```python
from build123d import *

# Parameters (mm, degrees)
F0_W     = 100
F0_H     = 100
F1_DEPTH = 50
F3_DEPTH = 25
F5_DEPTH = 22.275646797
F7_DEPTH = 100
F8_R     = 7.5
F8_W     = 10
F8_H     = 10
F9_DEPTH = 25
F9_TAPER = 3
F10_R    = 2
F11_R    = 0.5
F12_R    = 0.5


with BuildPart() as f1:
    # F0 (on Top) → F1 (new body)
    with BuildSketch(Plane.XY):
        Rectangle(F0_W, F0_H)
    extrude(amount=F1_DEPTH)

    # F2 (on face) → F3 (cut)
    with BuildSketch(Plane.XY.offset(50)):
        with BuildLine():
            ThreePointArc((-27.6920917798, 27.7259293121), (-31.8171440994, 25.5516150722), (-32.3544992545, 20.9196664012))
            add(Edge.make_bspline(
                [(-32.3544992545, 20.9196664012), (-23.103090057, -2.9601436233), (-0.2425590805, -61.5865364676), (23.6450097648, -2.9646096828), (32.5238265853, 20.9872745586)],
                knots=[0.0444691943, 0.0444691943, 0.0444691943, 0.0444691943, 0.5000014683, 0.9560875796, 0.9560875796, 0.9560875796, 0.9560875796], degree=3))
            ThreePointArc((32.5238265853, 20.9872745586), (31.9398334839, 25.5808897558), (27.8356444162, 27.7251799922))
            Line((27.8356444162, 27.7251799922), (-27.6920917798, 27.7259293121))
        make_face()
    extrude(amount=-F3_DEPTH, mode=Mode.SUBTRACT)

    # F4 (on face) → F5 (cut, through all)
    with BuildSketch(Plane(origin=(0, 50, 0), x_dir=(-1, 0, 0), z_dir=(0, 1, 0))):
        Polygon((15, 50), (-15, 50), (-12.5, 40), (12.5, 40), align=None)
    extrude(amount=-F5_DEPTH, mode=Mode.SUBTRACT)

    # F6 (on face) → F7 (cut)
    with BuildSketch(Plane(origin=(-50, 0, 0), x_dir=(0, -1, 0), z_dir=(-1, 0, 0))):
        Polygon((15, 50), (-15, 50), (-12.5, 40), (12.5, 40), align=None)
    extrude(amount=-F7_DEPTH, mode=Mode.SUBTRACT)

    # F8 (on face) → F9 (join)
    with BuildSketch(Plane.XY.offset(25)):
        Circle(F8_R)
        with Locations((16.3814044744, 15.9227793291)):
            Rectangle(F8_W, F8_H)
    extrude(amount=F9_DEPTH, taper=F9_TAPER)

    # F10
    f10_edges = [f1.edges().sort_by_distance(p)[0] for p in [
        (0.071776, 27.725555, 25),
        (31.939833, 25.58089, 25),
        (-31.817144, 25.551615, 25),
        (0.102186, -32.273864, 25),
        (-7.5, 0, 25),
        (11.381404, 15.922779, 25),
        (16.381404, 10.922779, 25),
        (21.381404, 15.922779, 25),
        (16.381404, 20.922779, 25),
    ]]
    fillet(f10_edges, radius=F10_R)

    # F11
    f11_edges = [f1.edges().sort_by_distance(p)[0] for p in [
        (-6.189806, 0, 50),
    ]]
    fillet(f11_edges, radius=F11_R)

    # F12
    f12_edges = [f1.edges().sort_by_distance(p)[0] for p in [
        (16.381404, 12.232974, 50),
        (12.691599, 15.922779, 50),
        (16.381404, 19.612585, 50),
        (20.07121, 15.922779, 50),
    ]]
    fillet(f12_edges, radius=F12_R)


solid = f1.part
```
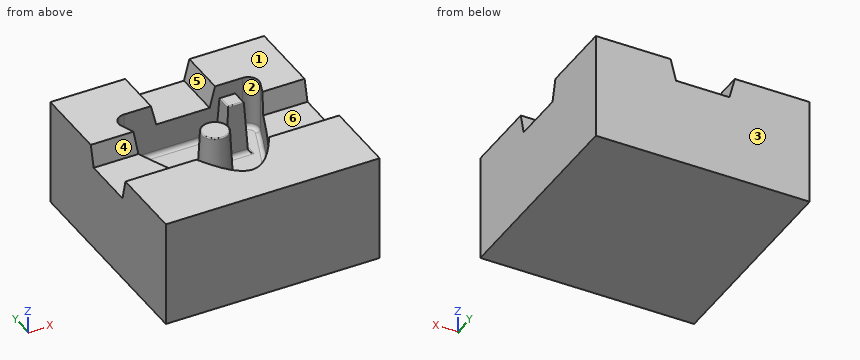
Verification items for the finished model (mm, model axes). Face numbers are marked on the shaded views. A direction names the side the tool comes from. Coordinates: 2 decimals unless noted, no trailing zeros. Answer as a JSON object with one key per item and string values.
(1) Go/stop test with flat-tipped pins: pin 1 Ø3 at (x, y) = (14.5, -4) entering from +Z; pin 2 Ø6.5 at (x, y) = (3.5, 41) entering from +Z. Record where each tip stops, or that it passes through.
Response:
{"pin 1": "stops at z = 25", "pin 2": "stops at z = 40"}
(2) Cross-section at A-A, the plane z = 28.5. Count the separate pieces of the cut face and the enclosed holes in it, then the cut area to 3 significant figures.
Response:
{"separate pieces": "3", "enclosed holes": "1", "area": "7,640 mm²"}
(3) Mould release check, pull along Y, two halves, no side actions. Record for the marked faces 1, 2 and 3: pulls with the +Y half, pulls with the -Y half, needs draft (parallel to the pull), parting line crosses it, or undercut.
Response:
{"face 1": "needs draft", "face 2": "undercut", "face 3": "pulls with the +Y half"}
(4) Scan lines: line 1 along Y through (x, z) = (13, 37.5); line 2 along Y through (x, z) = (-45, 44); line 3 along Z through (x, y) = (-8, -24.5). Record each from-to range of solid material in increasing order.
Response:
{"line 1": "y = -50 to -21.88, 11.58 to 20.27, 27.73 to 50", "line 2": "y = -50 to -13.5, 13.5 to 50", "line 3": "z = 0 to 25"}
(5) Access from +Z, -Z, +X, -X, +Y, -Y to the whole of each face (thin tool, end or side, straight path). Record for the marked faces 4, 5 and 6.
Response:
{"face 4": "+Z, -X", "face 5": "+Z, +Y", "face 6": "+Z, +X"}
